For this review, use the dimensioned drawing (mm, ordinates from the lowest corner) and the shaded views. Give positions to 0.01 mm unless a question says otherwise; leave off trailing zeros. Order: outer loops, then holes, each group sorted by start corner. A loop starts at its lowest first (then second) coordinate and runs counter-clockwise, first axis right, second up. Notation, with made-up numbers: (52, 43) - (75, 43) arc R26 cw to (75, 71) - close; hole circle Ø5 at (0, -13.75). An arc over 180 degrees is marked (long way). Use a Markdown table: item, result. Add a question column.
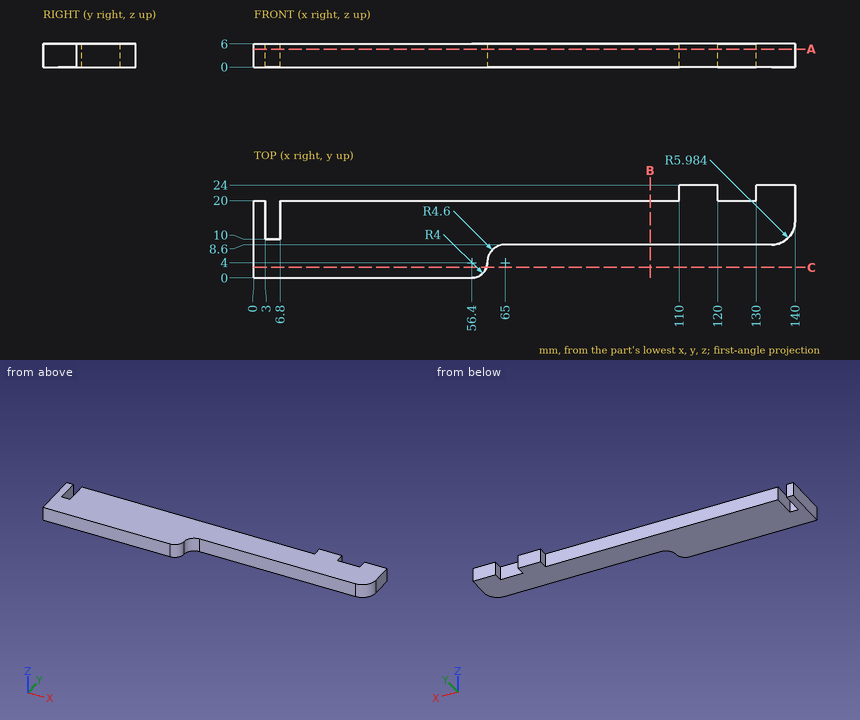
Q1. Clearance check with flat-ended pins moving along their axes: P1, Ø0.9, axis at x = 1.5, z = 1.5, coming from the +Y side; P2, Ø3, axis at y = 22.5, z = 2, coming from the -X side; P3, Ø1.1, axis at x = 4.5, z = 2, coming from the +Y side. State where each tip first meets the part, or that it passes through.
Q2. Wall thickness on probe 1 along X at (y, z) = (15.5, 4.25); probe 2 along Y at (x, z) = (105.5, 3.7); probe 3 along X at (y, z) = (10.5, 3.1): over which ranges is each line inside the solid? List them lowest first.
Q3. We need section C-C (y = 2.75). Write out the cut boundary in (x, z), plus the area to 3 significant figures.
Q4. We need section B-B (x = 102.5). Write out the cut boundary in (y, z).
Q5. We need section A-A (z = 4.65). Write out the cut boundary in (x, y).
Here are the results:
| question | item | result |
|---|---|---|
| 1 | P1 | y = 20 |
| 1 | P2 | x = 110 |
| 1 | P3 | y = 10 |
| 2 | probe 1 | 0 to 3, 6.8 to 140 |
| 2 | probe 2 | 8.6 to 20 |
| 2 | probe 3 | 0 to 3, 6.8 to 138.39 |
| 3 | outline | (0, 0) - (60.2, 0) - (60.2, 6) - (0, 6) - close |
| 3 | area | 361 mm2 |
| 4 | outline | (8.6, 0) - (20, 0) - (20, 6) - (8.6, 6) - close |
| 5 | outline | (0, 0) - (56.4, 0) arc R4 ccw to (60.4, 4) arc R4.6 cw to (65, 8.6) - (134.02, 8.6) arc R5.98 ccw to (140, 14.58) - (140, 24) - (130, 24) - (130, 20) - (120, 20) - (120, 24) - (110, 24) - (110, 20) - (6.8, 20) - (6.8, 10) - (3, 10) - (3, 20) - (0, 20) - close |
